Study the drawing (mm; zero at the part's minimum x, y, z) and answer. A direction names the side the tool comes from. Give positions to 0.01 mm unless a question says otherwise; leave off trailing zeros. Write each loop counter-clockwise with the first axis right and the second up, starting at its lowest first coordinate (ties: lowest second). Pieces come first, ordered by that corner, then holes.
1) A tool of negligible diameter and unlimited length cuts with its end or side. For the marked faces 1 and 2, from which of +Z, -Z, +X, -X, +Y, -Y can it reach the whole face along a straight path? Write none if from no direction.
2) Find section C-C (z = 34.9). Determine the outline of the cut face in (x, y).
3) Find section A-A (z = 23.9). Determine the outline of the cut face in (x, y).
4) Find section B-B (x = 22). Determine the outline of the cut face in (y, z).
5) Find section D-D (y = 5.5). Determine the outline of the cut face in (x, z).
6) Straight lines are drawn through the part: probe 1 along Z at (x, y) = (30, 38.55); probe 2 along Z at (x, y) = (22, 39); probe 3 along X at (y, z) = (39.05, 12.9). For each, find the intervals that lie inside material, in ascending order.
7) Given pin 1 Ø5 at (x, y) = (34.5, 26.5) entering from +Z; pin 2 Ø20.5 at (x, z) = (33, 25) entering from -Y, each flat-ended and moving along its own axis, determine where each tip first touches the part or whether it passes through.
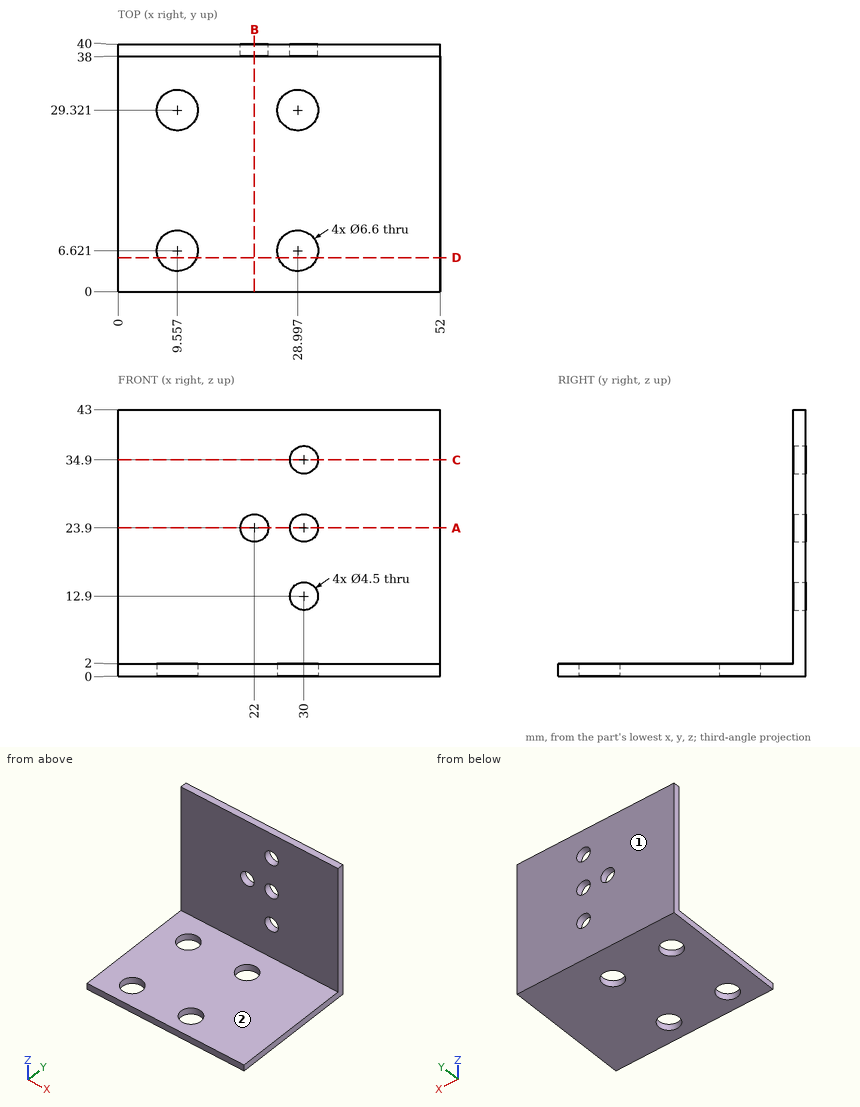
Results:
1. face 1: +Z, -Z, +X, -X, +Y
1. face 2: +Z, +X, -X, -Y
2. outline: (0, 38) - (27.75, 38) - (27.75, 40) - (0, 40) - close; (32.25, 38) - (52, 38) - (52, 40) - (32.25, 40) - close
3. outline: (0, 38) - (19.75, 38) - (19.75, 40) - (0, 40) - close; (24.25, 38) - (27.75, 38) - (27.75, 40) - (24.25, 40) - close; (32.25, 38) - (52, 38) - (52, 40) - (32.25, 40) - close
4. outline: (0, 0) - (40, 0) - (40, 21.65) - (38, 21.65) - (38, 2) - (0, 2) - close; (38, 26.15) - (40, 26.15) - (40, 43) - (38, 43) - close
5. outline: (0, 0) - (6.45, 0) - (6.45, 2) - (0, 2) - close; (12.66, 0) - (25.89, 0) - (25.89, 2) - (12.66, 2) - close; (32.1, 0) - (52, 0) - (52, 2) - (32.1, 2) - close
6. probe 1: z = 0 to 10.65, 15.15 to 21.65, 26.15 to 32.65, 37.15 to 43
6. probe 2: z = 0 to 21.65, 26.15 to 43
6. probe 3: x = 0 to 27.75, 32.25 to 52
7. pin 1: stops at z = 2
7. pin 2: stops at y = 38
